The listing builds one solid part. Answer for the finished solid, in the listing's coordinates (mm). A direction names the side the tool comes from. Give positions to 0.01 mm unless a question says otherwise; leave off trailing zeros. Loops run counter-clockwise (first coordinate to the right, second up) from the corner with the lowest first, then second, coordinate; pieces in that order, holes last. Notation, with made-up numbers: (-0.75, 71.5) - (58.25, 71.5) arc R20 ccw to (58.25, 99.5) - close; hole circle Ø3 at (49, -19). An arc over 180 degrees is marked (long way). Answer as CSV lines item,"result". Start each with the question number.
1) For a pull along Z with two mould halves and no side action, classify faces 6 (the face through (6, 9, -1.3)), 7 (the face through (4.214, 6, -1)), 8 (the face through (8.52, 0.125, 0.394)), 9 (the face through (4, 3, 0)) as pulls with the +Z half, pulls with the -Z half, needs draft (parallel to the pull), parting line crosses it, or undercut.
2) A cutting plane is placed at D-D (x = 4). Determine the outline of the cut face in (y, z), and give its area (3 significant figures).
3) A cutting plane is placed at A-A (z = -0.65). Determine the outline of the cut face in (x, y), and give its area (3 significant figures).
4) Find the intervals of material crossed by line 1 along X through (y, z) = (7, -1.2); line 2 along Z through (x, y) = (4.5, 7.75); line 3 along Z through (x, y) = (8, 1.25), in increasing order.
5) A cutting plane is placed at C-C (z = 0.45). Determine the outline of the cut face in (x, y), and give its area (3 significant figures).
6) For faces 1 (the face through (4, 3, -1.3)), 2 (the face through (9.662, 0.472, 0.394)), 3 (the face through (7.15, 0.14, 0.39)), 4 (the face through (5.158, 2.946, 0.394)), 5 (the face through (11.383, 7, -1)), determine the directions among +Z, -Z, +X, -X, +Y, -Y from which every point of the face is accessible in a straight line to the end or side of a thin tool.
7) A cutting plane is placed at B-B (y = 11.5). Determine the outline of the cut face in (x, z).
8) Flat-ended cylindrical pins translate along their axes: pin 1 (2 mm diameter, centred on x = 4.5, y = 1.5, fed in from +Z); pin 2 (1.5 mm diameter, centred on x = 6.5, z = -0.5, fed in from -Y). Find the tip coordinate at first contact, or state that the pin passes through.
```python
from build123d import *

# Parameters (mm, degrees)
BOSS_EXTRUDE1_DEPTH   = 0.8
SKETCH5_W             = 1
SKETCH5_H             = 13
SKETCH5_W_2           = 1.031823626
SKETCH5_H_2           = 8
BOSS_EXTRUDE2_DEPTH   = 1.3
BOSS_EXTRUDE3_DEPTH   = 0.8
M3_TAPPED_HOLE1_D     = 2.5
M3_TAPPED_HOLE1_DEPTH = 0.8
THREAD2_PITCH         = 0.5
CUT_EXTRUDE1_REACH    = 17.709
SKETCH12_R            = 0.3
CUT_EXTRUDE2_REACH    = 19.895
CUT_EXTRUDE3_REACH    = 17.709
SKETCH14_R            = 0.15


with BuildPart() as part:
    # Sketch1 → Boss-Extrude1 (new body)
    with BuildSketch(Plane.XY):
        Polygon((3.214446547, 12.558271664), (12.414446547, 12.558271664), (12.414446547, 4.558271664), (8.603545102, 1.360545667), (10.75141162, -0.441728336), (9.195687793, -0.441728336), (7.825683188, 0.707842022), (6.455678584, -0.441728336), (4.899954757, -0.441728336), (7.047821275, 1.360545667), (3.214446547, 4.577128987), align=None)
    extrude(amount=BOSS_EXTRUDE1_DEPTH)

    # Sketch5 → Boss-Extrude2 (add)
    with BuildSketch(Plane(origin=(0, 0, 0), x_dir=(-1, 0, 0), z_dir=(0, 0, -1))):
        with Locations((-3.714446547, 6.058271664)):
            Rectangle(SKETCH5_W, SKETCH5_H)
        with Locations((-11.898534734, 8.558271664)):
            Rectangle(SKETCH5_W_2, SKETCH5_H_2)
    extrude(amount=BOSS_EXTRUDE2_DEPTH)

    # Sketch8 → Boss-Extrude3 (add)
    with BuildSketch(Plane(origin=(0, 0, -1.3), x_dir=(-1, 0, 0), z_dir=(0, 0, -1))):
        Polygon((-12.414446547, 12.558271664), (-3.214446547, 12.558271664), (-3.214446547, 4.872903055), (-11.382622921, 4.872903055), (-11.382622921, -0.60025791), (-12.414446547, -0.60025791), align=None)
    extrude(amount=BOSS_EXTRUDE3_DEPTH)

    # M3 Tapped Hole1
    with Locations(Plane(origin=(0, 0, -1.3), x_dir=(-1, 0, 0), z_dir=(0, 0, 1))):
        with Locations((-7.814446547, -8.649654686)):
            Hole(M3_TAPPED_HOLE1_D / 2, depth=M3_TAPPED_HOLE1_DEPTH)

    # Thread2: the profile of Thread Profile4 profile screwed along a right-hand helix of 1.6 turns, 6 arcs to a turn; built about Z, then put on its axis
    thread2_z = Axis((0, 0, 0), (0, 0, 1))
    thread2_corners = [(1.2497, 0, -0.000173205), (1.520632937, 0, 0.156249999), (1.520632937, 0, 0.218749999), (1.2497, 0, 0.375173204)]
    with BuildLine(mode=Mode.PRIVATE) as thread2_profile:
        Line(thread2_corners[0], thread2_corners[1])
        Line(thread2_corners[1], thread2_corners[2])
        Line(thread2_corners[2], thread2_corners[3])
        Line(thread2_corners[3], thread2_corners[0])
    thread2_cap = Face(thread2_profile.wire())
    thread2_turn_angles = [0, 30, 60, 90, 120, 150, 180, 210, 240, 270, 300, 330, 360]
    thread2_turn_weights = [1, 0.8660254037844387, 1, 0.8660254037844387, 1, 0.8660254037844387, 1, 0.8660254037844387, 1, 0.8660254037844387, 1, 0.8660254037844387, 1]
    thread2_turn_rails = [Edge.make_bspline([Vector(p[0], p[1], 0).rotate(thread2_z, thread2_turn_angles[k]) / thread2_turn_weights[k] + Vector(0, 0, p[2] + THREAD2_PITCH * thread2_turn_angles[k] / 360) for k in range(13)], [0, 0, 0, 1, 1, 2, 2, 3, 3, 4, 4, 5, 5, 6, 6, 6], 2, thread2_turn_weights) for p in thread2_corners]
    thread2_turn_sides = [Face.make_surface_from_curves(thread2_turn_rails[p[0]], thread2_turn_rails[p[1]]) for p in [(0, 1), (1, 2), (2, 3), (3, 0)]]
    thread2_last_angles = [360, 390, 420, 450, 480, 510, 540, 558, 576]
    thread2_last_weights = [1, 0.8660254037844387, 1, 0.8660254037844387, 1, 0.8660254037844387, 1, 0.9510565162951535, 1]
    thread2_last_rails = [Edge.make_bspline([Vector(p[0], p[1], 0).rotate(thread2_z, thread2_last_angles[k]) / thread2_last_weights[k] + Vector(0, 0, p[2] + THREAD2_PITCH * thread2_last_angles[k] / 360) for k in range(9)], [0, 0, 0, 1, 1, 2, 2, 3, 3, 4, 4, 4], 2, thread2_last_weights) for p in thread2_corners]
    thread2_last_sides = [Face.make_surface_from_curves(thread2_last_rails[p[0]], thread2_last_rails[p[1]]) for p in [(0, 1), (1, 2), (2, 3), (3, 0)]]
    thread2 = Plane(origin=(7.814446547, 8.649654686, -2.1), x_dir=(1, 0, 0), z_dir=(0, 0, 1)) * Solid(Shell([*thread2_turn_sides, *thread2_last_sides, thread2_cap, thread2_cap.rotate(thread2_z, 576).moved(Location((0, 0, THREAD2_PITCH * 576 / 360)))]))
    add(thread2, mode=Mode.SUBTRACT)

    # Sketch12 → Cut-Extrude1 (cut, up to next)
    with BuildSketch(Plane.ZY.offset(-3.214446547), mode=Mode.PRIVATE) as cut_extrude1_sk1:
        with Locations(Location((-0.65, 1.055227185, 0), (0, 0, 270))):
            Circle(SKETCH12_R)
    cut_extrude1_tool1 = extrude(cut_extrude1_sk1.sketch, amount=-CUT_EXTRUDE1_REACH, mode=Mode.PRIVATE) & part.part
    # Sketch12 → Cut-Extrude1 (cut, up to next)
    with BuildSketch(Plane.ZY.offset(-3.214446547), mode=Mode.PRIVATE) as cut_extrude1_sk2:
        Polygon((-1.3, 0.491189657), (-1, -0.121721645), (-1.3, -0.121721645), align=None)
    cut_extrude1_tool2 = extrude(cut_extrude1_sk2.sketch, amount=-CUT_EXTRUDE1_REACH, mode=Mode.PRIVATE) & part.part
    # Sketch12 → Cut-Extrude1 (cut, up to next)
    with BuildSketch(Plane.ZY.offset(-3.214446547), mode=Mode.PRIVATE) as cut_extrude1_sk3:
        Polygon((0, 0.491189657), (-0.3, -0.121721645), (0, -0.121721645), align=None)
    cut_extrude1_tool3 = extrude(cut_extrude1_sk3.sketch, amount=-CUT_EXTRUDE1_REACH, mode=Mode.PRIVATE) & part.part
    add(cut_extrude1_tool1.solids().sort_by_distance((3.214447, 1.055227, -0.65))[0], mode=Mode.SUBTRACT)
    add(cut_extrude1_tool2.solids().sort_by_distance((3.214447, 0.082582, -1.2))[0], mode=Mode.SUBTRACT)
    add(cut_extrude1_tool3.solids().sort_by_distance((3.214447, 0.082582, -0.1))[0], mode=Mode.SUBTRACT)

    # Sketch13 → Cut-Extrude2 (cut, up to next)
    with BuildSketch(Plane.XY.offset(0.8), mode=Mode.PRIVATE) as cut_extrude2_sk1:
        Polygon((4.634176401, 6.767991384), (4.634176401, 5.073282991), (7.825683188, 2.395290823), (10.687148853, 4.796345607), (10.687148853, 8.674644795), align=None)
    cut_extrude2_tool1 = extrude(cut_extrude2_sk1.sketch, amount=-CUT_EXTRUDE2_REACH, mode=Mode.PRIVATE) & part.part
    add(cut_extrude2_tool1.solids().sort_by_distance((7.949639, 5.66496, 0.8))[0], mode=Mode.SUBTRACT)

    # Sketch14 → Cut-Extrude3 (cut, up to next)
    with BuildSketch(Plane(origin=(12.414446547, 0, 0), x_dir=(0, 0, -1), z_dir=(1, 0, 0)), mode=Mode.PRIVATE) as cut_extrude3_sk1:
        with Locations(Location((1.8, 0.598886989, 0), (0, 0, 90))):
            Circle(SKETCH14_R)
    cut_extrude3_tool1 = extrude(cut_extrude3_sk1.sketch, amount=-CUT_EXTRUDE3_REACH, mode=Mode.PRIVATE) & part.part
    # Sketch14 → Cut-Extrude3 (cut, up to next)
    with BuildSketch(Plane(origin=(12.414446547, 0, 0), x_dir=(0, 0, -1), z_dir=(1, 0, 0)), mode=Mode.PRIVATE) as cut_extrude3_sk2:
        Polygon((1.3, 0.13596653), (1.5, -0.371538896), (1.3, -0.371538896), align=None)
    cut_extrude3_tool2 = extrude(cut_extrude3_sk2.sketch, amount=-CUT_EXTRUDE3_REACH, mode=Mode.PRIVATE) & part.part
    # Sketch14 → Cut-Extrude3 (cut, up to next)
    with BuildSketch(Plane(origin=(12.414446547, 0, 0), x_dir=(0, 0, -1), z_dir=(1, 0, 0)), mode=Mode.PRIVATE) as cut_extrude3_sk3:
        Polygon((2.1, 0.13596653), (1.9, -0.371538896), (2.1, -0.371538896), align=None)
    cut_extrude3_tool3 = extrude(cut_extrude3_sk3.sketch, amount=-CUT_EXTRUDE3_REACH, mode=Mode.PRIVATE) & part.part
    add(cut_extrude3_tool1.solids().sort_by_distance((12.414447, 0.598887, -1.8))[0], mode=Mode.SUBTRACT)
    add(cut_extrude3_tool2.solids().sort_by_distance((12.414447, -0.20237, -1.366667))[0], mode=Mode.SUBTRACT)
    add(cut_extrude3_tool3.solids().sort_by_distance((12.414447, -0.20237, -2.033333))[0], mode=Mode.SUBTRACT)


solid = part.part
```
Ans:
1,face 6,"undercut"
1,face 7,"undercut"
1,face 8,"needs draft"
1,face 9,"pulls with the +Z half"
2,outline,"(-0.44, -1.3) - (-0.12, -1.3) - (-0.12, -1) - (0.49, -1.3) - (4.87, -1.3) - (4.87, -2.1) - (12.56, -2.1) - (12.56, 0.8) - (3.92, 0.8) - (3.92, 0) - (0.49, 0) - (-0.12, -0.3) - (-0.12, 0) - (-0.44, 0) - close; hole circle Ø0.6 at (1.06, -0.65)"
2,area,"29.5 mm2"
3,outline,"(3.21, -0.44) - (4.21, -0.44) - (4.21, 0.76) - (3.21, 0.76) - close; (3.21, 1.36) - (4.21, 1.36) - (4.21, 12.56) - (3.21, 12.56) - close; (11.38, 4.56) - (12.41, 4.56) - (12.41, 12.56) - (11.38, 12.56) - close"
3,area,"20.7 mm2"
4,line 1,"3.21 to 4.21, 11.38 to 12.41"
4,line 2,"-2.1 to -1.3, 0 to 0.8"
4,line 3,"0 to 0.8"
5,outline,"(3.21, 4.58) - (7.05, 1.36) - (4.9, -0.44) - (6.46, -0.44) - (7.83, 0.71) - (9.2, -0.44) - (10.75, -0.44) - (8.6, 1.36) - (12.41, 4.56) - (12.41, 12.56) - (3.21, 12.56) - close; hole (4.63, 5.07) - (7.83, 2.4) - (10.69, 4.8) - (10.69, 8.67) - (4.63, 6.77) - close"
5,area,"71.3 mm2"
6,face 1,"-Z, -X, -Y"
6,face 2,"+Z, -Z, +X"
6,face 3,"+Z, -Z, -Y"
6,face 4,"+Z, -X"
6,face 5,"-Y"
7,outline,"(3.21, -2.1) - (12.41, -2.1) - (12.41, 0.8) - (3.21, 0.8) - close; hole (4.21, -1.3) - (11.38, -1.3) - (11.38, 0) - (4.21, 0) - close"
8,pin 1,"z = 0"
8,pin 2,"y = -0.44"
